Could you check a few things on this model? Use its own coordinates, in mm. Round coordinates to 2 decimals unless told otherwise and drop trailing zeros. Loops run counter-clockwise (first coordinate to the right, second up) from the corner with the lowest first, then second, coordinate; pieces in that order, holes last.
from build123d import *

# Parameters (mm, degrees)
SKETCH1_W           = 100
SKETCH1_H           = 50
SKETCH1_R           = 7.5
BOSS_EXTRUDE1_DEPTH = 10
CUT_EXTRUDE1_DEPTH  = 5


with BuildPart() as part:
    # Sketch1 → Boss-Extrude1 (new body)
    with BuildSketch(Plane.XY):
        with Locations((50, 25)):
            Rectangle(SKETCH1_W, SKETCH1_H)
        with Locations((87.5, 37.5)):
            Circle(SKETCH1_R, mode=Mode.SUBTRACT)
    extrude(amount=BOSS_EXTRUDE1_DEPTH)

    # Sketch2 → Cut-Extrude1 (cut)
    with BuildSketch(Plane.XY.offset(10)):
        Polygon((25.773502692, 25), (14.226497308, 25), (8.452994616, 15), (14.226497308, 5), (25.773502692, 5), (31.547005384, 15), align=None)
    cut_extrude1 = extrude(amount=-CUT_EXTRUDE1_DEPTH, mode=Mode.SUBTRACT)

    # Mirror1: Cut-Extrude1 across plane
    add(cut_extrude1.mirror(Plane.ZY.offset(-50)), mode=Mode.SUBTRACT)

    # Mirror3: part across plane


with BuildPart() as part_1:
    add(part.part)
    add(part.part.mirror(Plane(origin=(0, 0, 10), x_dir=(0, 0, 1), z_dir=(0, 1, 0))))

    # Mirror4: part across plane


with BuildPart() as part_2:
    add(part_1.part)
    add(part_1.part.mirror(Plane(origin=(100, 0, 10), x_dir=(0, 0, 1), z_dir=(-1, 0, 0))))

    # Mirror5: part across plane


with BuildPart() as part_3:
    add(part_2.part)
    add(part_2.part.mirror(Plane(origin=(0, 0, 0), x_dir=(1, 0, 0), z_dir=(0, 0, -1))))


solid = part_3.part
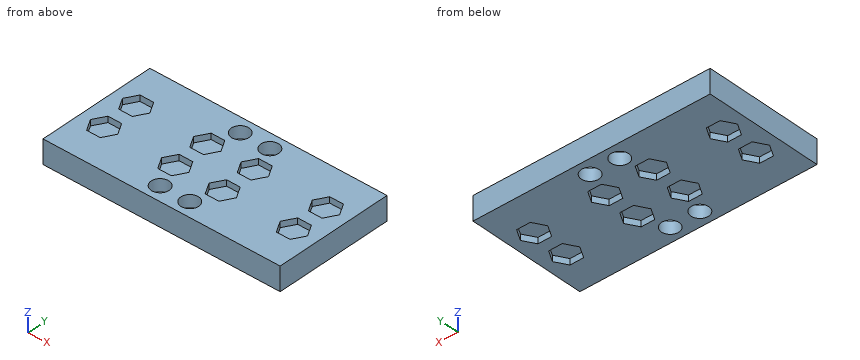
Item 1: If I drill on line 1 along X through (y, z) = (37, 8.5); line 2 along X through (y, z) = (36.5, 6); line 3 along X through (y, z) = (-20.5, 7.5), over which ranges is the centre line in solid material (lowest first)?
Results list:
line 1: x = 0 to 80.02, 94.98 to 105.02, 119.98 to 200
line 2: x = 0 to 80.07, 94.93 to 105.07, 119.93 to 200
line 3: x = 0 to 11.63, 28.37 to 71.63, 88.37 to 111.63, 128.37 to 171.63, 188.37 to 200
Item 2: If we section it at B-B, the plane x = 123.5: Please give me the cut outline in (y, z).
Results list:
outline: (-50, -10) - (-25, -10) - (-25, -5) - (-5, -5) - (-5, -10) - (5, -10) - (5, -5) - (25, -5) - (25, -10) - (50, -10) - (50, 10) - (25, 10) - (25, 5) - (5, 5) - (5, 10) - (-5, 10) - (-5, 5) - (-25, 5) - (-25, 10) - (-50, 10) - close
Item 3: If we section it at D-D, the plane y = 39.5: Please give me the cut outline in (x, z).
Results list:
outline: (0, -10) - (80.27, -10) - (80.27, 10) - (0, 10) - close; (94.73, -10) - (105.27, -10) - (105.27, 10) - (94.73, 10) - close; (119.73, -10) - (200, -10) - (200, 10) - (119.73, 10) - close
Item 4: If we section it at C-C, the plane z = -7: Count the separate pieces of the cut face and the enclosed holes in it, then the cut area to 3 significant figures.
Results list:
separate pieces: 1
enclosed holes: 12
area: 16,500 mm2
Item 5: Will these pins go through, and if not, where does the flat tip stop? pin 1 (6 mm diameter, centred on x = 22.5, y = 19.5, fed in from -Z); pin 2 (16 mm diameter, centred on x = 82, y = -15, fed in from +Z); pin 3 (9 mm diameter, centred on x = 112.5, y = -37.5, fed in from +Z).
Results list:
pin 1: stops at z = -5
pin 2: stops at z = 5
pin 3: passes through
Item 6: If we section it at A-A, the plane y = -37.5: Please give me the cut outline in (x, z), then the cut area to 3 significant figures.
Results list:
outline: (0, -10) - (80, -10) - (80, 10) - (0, 10) - close; (95, -10) - (105, -10) - (105, 10) - (95, 10) - close; (120, -10) - (200, -10) - (200, 10) - (120, 10) - close
area: 3,400 mm2
